```python
from build123d import *

# Parameters (mm, degrees)
F0_W     = 100.3
F0_H     = 170.3
F1_DEPTH = 1.5
F0_W_2   = 103.3
F0_H_2   = 173.3
F2_DEPTH = 15
F3_R     = 5
F4_W     = 15
F4_H     = 10
F5_DEPTH = 25


with BuildPart() as f1:
    # F0 (on Top) → F1 (new body)
    with BuildSketch(Plane.XY):
        with Locations((50.15, -85.15)):
            Rectangle(F0_W, F0_H)
    extrude(amount=F1_DEPTH)

    # F0 (on Top) → F2 (join)
    with BuildSketch(Plane.XY):
        with Locations((50.15, -85.15)):
            Rectangle(F0_W_2, F0_H_2)
        with Locations((50.15, -85.15)):
            Rectangle(F0_W, F0_H, mode=Mode.SUBTRACT)
    extrude(amount=F2_DEPTH)

    # F3
    f3_edges = [f1.edges().sort_by_distance(p)[0] for p in [
        (0, 0, 8.25),
        (101.8, 1.5, 7.5),
        (100.3, 0, 8.25),
        (-1.5, 1.5, 7.5),
        (100.3, -170.3, 8.25),
        (-1.5, -171.8, 7.5),
        (0, -170.3, 8.25),
        (101.8, -171.8, 7.5),
        (50.15, 1.5, 0),
        (-1.5, -85.15, 0),
        (50.15, -171.8, 0),
        (101.8, -85.15, 0),
        (50.15, 0, 1.5),
        (0, -85.15, 1.5),
        (50.15, -170.3, 1.5),
        (100.3, -85.15, 1.5),
    ]]
    fillet(f3_edges, radius=F3_R)

    # F4 (on face) → F5 (cut)
    with BuildSketch(Plane(origin=(0, 0, 0), x_dir=(1, 0, 0), z_dir=(0, 0, -1))):
        with Locations((16, 161.8)):
            Rectangle(F4_W, F4_H)
    extrude(amount=-F5_DEPTH, mode=Mode.SUBTRACT)


solid = f1.part
```
Part model, mm, in its own coordinate system. A direction names the side the tool comes from. Round coordinates to 2 decimals unless told otherwise and drop trailing zeros. Order: outer loops, then holes, each group sorted by start corner. A loop starts at its lowest first (then second) coordinate and runs counter-clockwise, first axis right, second up. Notation, with made-up numbers: M 68.25,56 L 122.25,56 A18 ccw 122.25,75 Z; hole C -27.75,34.25 d9. An arc over 180 degrees is marked long. Put each result on its own line as item: value. Start each with the question number.
1. Slice it at A-A on x = 20.5. List the corners of the cut face in (y, z), then the cut area to 3 significant figures.
2. Slice it at D-D on y = -91. List the corners of the cut face in (x, z), then the cut area to 3 significant figures.
3. Slice it at C-C on x = 42. List the corners of the cut face in (y, z), then the cut area to 3 significant figures.
4. Drill centre lines: probe 1 along X at (y, z) = (-161.5, 11.75); probe 2 along Y at (x, z) = (10.5, 13); probe 3 along Z at (x, y) = (43.5, -75.5). Where is each one in solid material? Low to high. Write a range as [from, to].
5. Two-plate mould, pull along X, no slides. Class faces 1 (the face through (0, -86, 11)), 2 (the face through (-0.07, 0, 10.07)), 3 (the face through (49, -171.8, 10)): +X half, -X half, draft (parallel to the pull), parting line (faces both ways), or undercut.
6. Slice it at B-B on z = 9.25. List the corners of the cut face in (x, y), then the cut area to 3 significant figures.
7. Drop flat-ended pins along their axis: pin 1 (1.9 mm diameter, centred on y = -162, z = 1, fed in from +X); pin 2 (0.5 mm diameter, centred on y = -162.5, z = 1.5, fed in from -X); pin 3 (1.9 mm diameter, centred on x = 15.5, z = 1, fed in from +Y). Give the stop position or say it passes through.
8. Tool access for faces 4 (the face through (50.78, -1.43, 3)), 5 (the face through (49, -84, 0)): list every direction of +Z, -Z, +X, -X, +Y, -Y with a clear straight run to the whole face (end or side of a thin tool).
Findings:
1. outline: M -171.8,5 A5 ccw -166.8,0 L -166.8,1.73 A5 cw -170.3,6.5 L -170.3,15 L -171.8,15 Z; M -156.8,0 L -3.5,0 A5 ccw 1.5,5 L 1.5,15 L 0,15 L 0,6.5 A5 cw -5,1.5 L -156.8,1.5 Z
1. area: 285 mm2
2. outline: M -1.5,5 A5 ccw 3.5,0 L 96.8,0 A5 ccw 101.8,5 L 101.8,15 L 100.3,15 L 100.3,6.5 A5 cw 95.3,1.5 L 5,1.5 A5 cw 0,6.5 L 0,15 L -1.5,15 Z
2. area: 195 mm2
3. outline: M -171.8,5 A5 ccw -166.8,0 L -3.5,0 A5 ccw 1.5,5 L 1.5,15 L 0,15 L 0,6.5 A5 cw -5,1.5 L -165.3,1.5 A5 cw -170.3,6.5 L -170.3,15 L -171.8,15 Z
3. area: 300 mm2
4. probe 1: [-1.5, 0], [100.3, 101.8]
4. probe 2: [-171.8, -170.3], [0, 1.5]
4. probe 3: [0, 1.5]
5. face 1: undercut
5. face 2: -X half
5. face 3: draft
6. outline: M -1.5,-166.8 A5 ccw 3.5,-171.8 L 96.8,-171.8 A5 ccw 101.8,-166.8 L 101.8,-3.5 A5 ccw 96.8,1.5 L 3.5,1.5 A5 ccw -1.5,-3.5 Z; hole M 0,-165.3 A5 ccw 5,-170.3 L 95.3,-170.3 A5 ccw 100.3,-165.3 L 100.3,-5 A5 ccw 95.3,0 L 5,0 A5 ccw 0,-5 Z
6. area: 821 mm2
7. pin 1: x = 100.76
7. pin 2: x = -0.3
7. pin 3: y = 0.46
8. face 4: +Z
8. face 5: -Z, +X, -X, +Y, -Y
